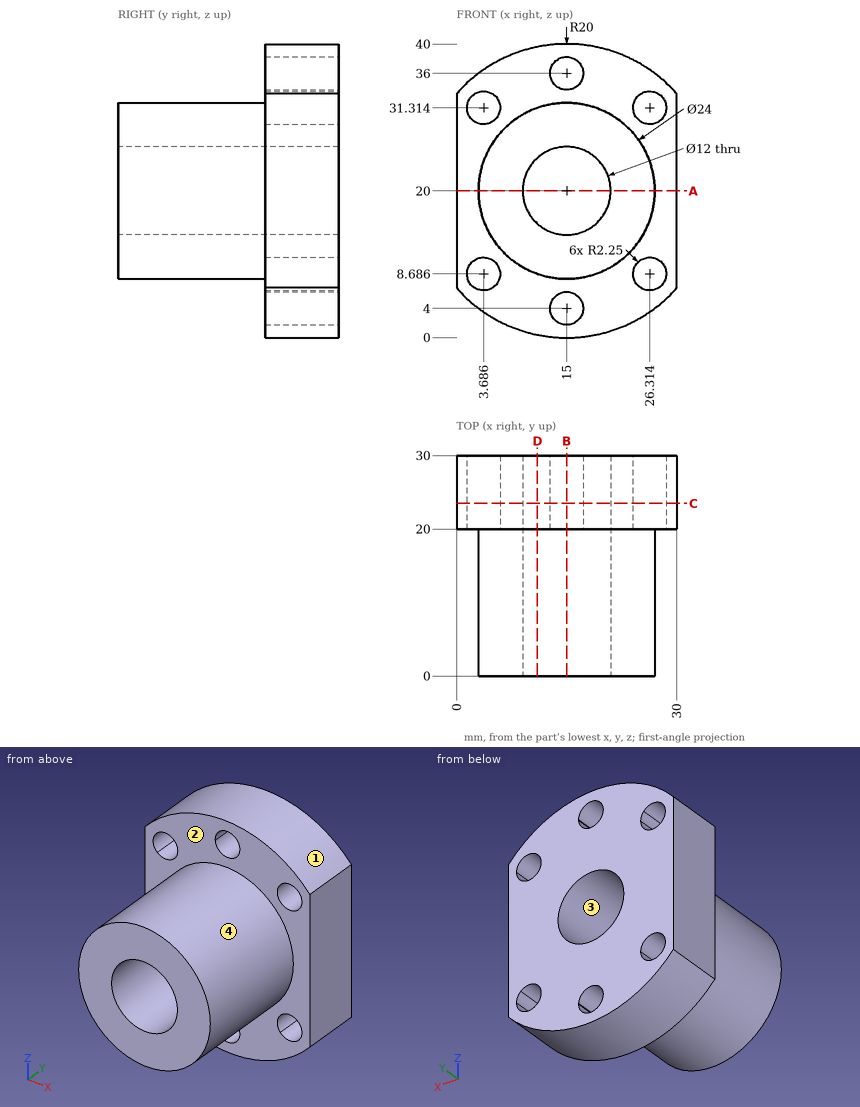
For this review, use the dimensioned drawing (mm, ordinates from the lowest corner) and the shaded views. Give positions to 0.01 mm unless a question says otherwise; leave off trailing zeros. Write each loop counter-clockwise with the first axis right and the second up, starting at its lowest first coordinate (ties: lowest second). Pieces come first, ordered by that corner, then holes. Notation, with made-up numbers: M 77.25,-19 L 101.25,-19 A27 ccw 101.25,1 Z; hole C 7,30.5 d1. An arc over 180 degrees is marked long. Answer as a JSON object with one key per item and string values. Group by question number.
Item 1: Consider section D-D on x = 11. Write out the cut boundary in (y, z).
Item 2: Consider section A-A on z = 20. Write out the cut boundary in (x, y), plus the area to 3 significant figures.
Item 3: For probe 1 along Z at (x, y) = (15, 22); probe 2 along Z at (x, y) = (15, 14.5); probe 3 along X at (y, z) = (24, 9) (1 decimal), list the stretches that pass through material, from the lowest coordinate up. Write a range as [from, to].
Item 4: For pin 1 Ø4 at (x, y) = (26, 20) entering from -Z; pin 2 Ø1.5 at (x, y) = (12.5, 18.5) entering from +Z; pin 3 Ø1 at (x, y) = (11.5, 22) entering from +Z, all flat-tipped, find the tip position at first contact; note any pin that passes through.
Item 5: Consider section B-B on x = 15. Write out the cut boundary in (y, z), plus the area to 3 significant figures.
Item 6: Consider section C-C on y = 23.5. Count the separate pieces of the cut face and the enclosed holes in it, plus the area to 3 significant figures.
Item 7: Draft analysis for pull direction Z (two halves, no side actions). For the marked faces 1, 2, 3 and 4, state which applies: +Z half, -Z half, draft (parallel to the pull), parting line (faces both ways), or undercut.
Check result:
{
 "1": {"outline": "M 0,8.69 L 20,8.69 L 20,0.4 L 30,0.4 L 30,15.53 L 0,15.53 Z; M 0,24.47 L 30,24.47 L 30,39.6 L 20,39.6 L 20,31.31 L 0,31.31 Z"},
 "2": {"outline": "M 0,20 L 3,20 L 3,0 L 9,0 L 9,30 L 0,30 Z; M 21,0 L 27,0 L 27,20 L 30,20 L 30,30 L 21,30 Z", "area": "420 mm^2"},
 "3": {"probe 1": "z = [0, 1.75], [6.25, 14], [26, 33.75], [38.25, 40]", "probe 2": "z = [8, 14], [26, 32]", "probe 3": "x = [0, 1.5], [5.9, 24.1], [28.5, 30]"},
 "4": {"pin 1": "stops at z = 2.14", "pin 2": "stops at z = 31.87", "pin 3": "stops at z = 39.77"},
 "5": {"outline": "M 0,8 L 20,8 L 20,6.25 L 30,6.25 L 30,14 L 0,14 Z; M 0,26 L 30,26 L 30,33.75 L 20,33.75 L 20,32 L 0,32 Z; M 20,0 L 30,0 L 30,1.75 L 20,1.75 Z; M 20,38.25 L 30,38.25 L 30,40 L 20,40 Z", "area": "430 mm^2"},
 "6": {"separate pieces": "1", "enclosed holes": "7", "area": "867 mm^2"},
 "7": {"face 1": "+Z half", "face 2": "draft", "face 3": "undercut", "face 4": "parting line"}
}
